from build123d import *

# Parameters (mm, degrees)
BOSS_EXTRUDE1_DEPTH = 22.5425
CUT_EXTRUDE1_DEPTH  = 14.605
SKETCH3_R           = 1.3462
CUT_EXTRUDE2_DEPTH  = 11.1125
SKETCH4_R           = 2.7305
CUT_EXTRUDE3_DEPTH  = 2.54
SCALE1_SCALE        = 0.6


with BuildPart() as part:
    # Sketch1 → Boss-Extrude1 (new, symmetric)
    with BuildSketch(Plane.XY):
        with BuildLine():
            Line((-77.49921, 0), (77.49921, 0))
            ThreePointArc((77.49921, 0), (83.25218384, -10.591022368), (71.236165373, -9.652))
            Line((71.236165373, -9.652), (65.40881, -9.652))
            Line((65.40881, -9.652), (65.40881, -5.4864))
            Line((65.40881, -5.4864), (71.663839849, -5.4864))
            ThreePointArc((71.663839849, -5.4864), (83.093360732, -9.011673362), (72.250559507, -3.9624))
            Line((72.250559507, -3.9624), (-72.250559507, -3.9624))
            ThreePointArc((-72.250559507, -3.9624), (-83.093360732, -9.011673362), (-71.663839849, -5.4864))
            Line((-71.663839849, -5.4864), (-65.40881, -5.4864))
            Line((-65.40881, -5.4864), (-65.40881, -9.652))
            Line((-65.40881, -9.652), (-71.236165373, -9.652))
            ThreePointArc((-71.236165373, -9.652), (-83.25218384, -10.591022368), (-77.49921, 0))
        make_face()
    extrude(amount=BOSS_EXTRUDE1_DEPTH, both=True)

    # Sketch2 → Cut-Extrude1 (cut)
    with BuildSketch(Plane(origin=(0, 0, 0), x_dir=(1, 0, 0), z_dir=(0, 1, 0))):
        with BuildLine():
            Line((84.35721, -14.5415), (84.35721, 14.5415))
            Line((84.35721, 14.5415), (21.2725, 14.5415))
            ThreePointArc((21.2725, 14.5415), (17.904903955, 13.146596045), (16.51, 9.779))
            Line((16.51, 9.779), (16.51, -9.779))
            ThreePointArc((16.51, -9.779), (17.904903955, -13.146596045), (21.2725, -14.5415))
            Line((21.2725, -14.5415), (84.35721, -14.5415))
        make_face()
        with BuildLine():
            Line((-84.35721, 14.5415), (-84.35721, -14.5415))
            Line((-84.35721, -14.5415), (-21.2725, -14.5415))
            ThreePointArc((-21.2725, -14.5415), (-17.904903955, -13.146596045), (-16.51, -9.779))
            Line((-16.51, -9.779), (-16.51, 9.779))
            ThreePointArc((-16.51, 9.779), (-17.904903955, 13.146596045), (-21.2725, 14.5415))
            Line((-21.2725, 14.5415), (-84.35721, 14.5415))
        make_face()
    extrude(amount=-CUT_EXTRUDE1_DEPTH, mode=Mode.SUBTRACT)

    # Sketch3 → Cut-Extrude2 (cut, symmetric)
    with BuildSketch(Plane.XZ.offset(9.652)):
        with Locations((68.322487686, 18.542)):
            Circle(SKETCH3_R)
        with Locations((68.322487686, -18.542)):
            Circle(SKETCH3_R)
        with Locations((-68.322487686, -18.542)):
            Circle(SKETCH3_R)
        with Locations(Location((-68.322487686, 18.542, 0), (0, 0, 270))):
            Circle(SKETCH3_R)
    extrude(amount=CUT_EXTRUDE2_DEPTH, both=True, mode=Mode.SUBTRACT)

    # Sketch4 → Cut-Extrude3 (cut)
    with BuildSketch(Plane(origin=(0, 0, 0), x_dir=(1, 0, 0), z_dir=(0, 1, 0))):
        with Locations(Location((-68.322487686, 18.542, 0), (0, 0, 180))):
            Circle(SKETCH4_R)
        with Locations(Location((-68.322487686, -18.542, 0), (0, 0, 180))):
            Circle(SKETCH4_R)
        with Locations(Location((68.322487686, -18.542, 0), (0, 0, 180))):
            Circle(SKETCH4_R)
        with Locations(Location((68.322487686, 18.542, 0), (0, 0, 180))):
            Circle(SKETCH4_R)
    extrude(amount=-CUT_EXTRUDE3_DEPTH, mode=Mode.SUBTRACT)


with BuildPart() as part_1:
    # Scale1: scaled about (0, -2.581706213, 0)
    add(part.part.scale(SCALE1_SCALE).moved(Location((0, -1.032682485, 0))))


solid = part_1.part
Can you work these out from the model? Positions are in its coordinate system, mm. A direction names the side the tool comes from. Round coordinates to 2 decimals unless told otherwise and drop trailing zeros. Loops run counter-clockwise (first coordinate to the right, second up) from the corner with the lowest first, then second, coordinate; pieces in that order, holes last. Notation, with made-up numbers: (68, 34) - (82, 34) arc R24 ccw to (82, 66) - close; hole circle Ø1 at (43, 42). An arc over 180 degrees is marked (long way). Write item = value, one per line. Start each with the question number.
(1) For faces 1 (the face through (-9.906, -2, 0)), 2 (the face through (9.906, -2, 0)), 3 (the face through (-42, -4.325, 11)), 4 (the face through (-40, -2.557, 11)), which set-ups out of +Z, -Z, +X, -X, +Y, -Y let a thin tool reach every point of the face, with its end or its side?
(2) If I drill on probe 1 along X at (y, z) = (-6.5, 10.75); probe 2 along Z at (x, y) = (12.5, -2.75); probe 3 along X at (y, z) = (-6.75, -11.75), over which ranges is the centre line in solid material (lowest first)? Write a range as [from, to].
(3) If we section it at C-C (x = -11): Please give me the cut outline in (y, z), and give its area (3 significant figures).
(4) For P1, Ø1.6, axis at x = -41, z = -11, coming from the +Y side; P2, Ø2.5, axis at x = -40.99, z = 11.13, coming from the -Y side; P3, Ø1, axis at y = -2.5, z = 10.5, coming from the -X side, each with a flat end and sliding along its axis, tell me the tip position at first contact or that it passes through.
(5) If we section it at A-A (x = 26): Please give me the cut outline in (y, z).
(6) If we mould it in two halves opening along Y, with no side actions, what happens to faces 5 (the face through (-39.8, -1.8, -10)), 6 (the face through (49.8, -6.58, -11.09)), 7 (the face through (50.02, -7.28, 11.16))? For each: released by +Y, released by -Y, zero draft, split by the parting line, or undercut.
(7) If we section it at B-B (z = 0): Please give me the cut outline in (x, y).
(8) If we section it at D-D (x = 5.5): Please give me the cut outline in (y, z).
Ans:
q1.face_1 = -X, +Y, -Y
q1.face_2 = +X, +Y, -Y
q1.face_3 = +Z, -Z
q1.face_4 = +Y
q2.probe_1 = [-50.39, -49.83], [-43.17, -41.71], [-40.28, -39.25], [39.25, 40.28], [41.71, 43.17], [49.83, 50.39]
q2.probe_2 = [-13.53, -8.71], [8.71, 13.53]
q2.probe_3 = [-50.29, -49.72], [-43.28, -41.51], [-40.48, -39.25], [39.25, 40.48], [41.51, 43.28], [49.72, 50.29]
q3.outline = (-3.41, -13.53) - (-1.03, -13.53) - (-1.03, -8.12) - (-3.41, -8.12) - close; (-3.41, 8.12) - (-1.03, 8.12) - (-1.03, 13.53) - (-3.41, 13.53) - close
q3.area = 25.7 mm²
q4.P1 = -2.56
q4.P2 = -6.82
q4.P3 = -50.01
q5.outline = (-3.41, -13.53) - (-1.03, -13.53) - (-1.03, -8.72) - (-3.41, -8.72) - close; (-3.41, 8.72) - (-1.03, 8.72) - (-1.03, 13.53) - (-3.41, 13.53) - close
q6.face_5 = zero draft
q6.face_6 = undercut
q6.face_7 = split by the parting line
q7.outline = (-9.91, -3.41) - (9.91, -3.41) - (9.91, -1.03) - (-9.91, -1.03) - close
q8.outline = (-3.41, -13.53) - (-1.03, -13.53) - (-1.03, 13.53) - (-3.41, 13.53) - close
